Input: dimensioned drawing with shaded views. Units: mm. Origin: part minimum x, y, z. A direction names the side the tool comes from. Round coordinates to 2 decimals unless told otherwise and drop trailing zeros. Order: outer loops, then holes, each group sorted by start corner. A loop starts at its lowest first (then second) coordinate and runs counter-clockwise, first axis right, second up. Notation, with made-up numbers: (-10, -15) - (22, -15) arc R21 ccw to (22, -1) - close; hole circle Ø2 at (49, -18.5). An arc over 180 degrees is marked (long way). Return JSON: item names as keys, results as strings. Group by question number.
1) Contact query for flat-ended pins moving along their axis: P1, Ø1.5, axis at x = 12.5, y = 4, coming from the +Z side; P2, Ø1, axis at x = 54.5, z = 8.5, coming from the -Y side; P3, Ø6, axis at y = 9.5, z = 5, coming from the +X side; P4, Ø7.5, axis at x = 13.5, z = 10, coming from the +Y side. Output: stop coordinate, or through.
2) Access query for the marked faces 4, 5, 6, 7 and 8. Directions: +Z, -Z, +X, -X, +Y, -Y. A direction counts if a zero-diameter tool reaches every point of the face in a straight line with its end or side. Return the directions, or none.
3) Section A-A, the plane x = 88.9. Return loops of the section in (y, z), plus the area to 3 significant figures.
4) Section B-B, the plane y = 3.75. Return loops of the section in (x, z), plus the area to 3 significant figures.
5) Section D-D, the plane x = 73. Return loops of the section in (y, z).
6) Section C-C, the plane z = 22.86. Return loops of the section in (x, y), plus the area to 3 significant figures.
7) Ray query, line 1 (X direction, y = 1, z = 2.54); line 2 (Z direction, x = 88.9, y = 0.9); line 3 (X direction, y = 3.75, z = 12.5). Return the intervals inside material, ascending. Write a range as from..to.
8) Mould query, pull axis X, two halves, no side actions, for the marked faces 1, 2 and 3. Classes: pulls with the +X half, pulls with the -X half, needs draft (parallel to the pull), parting line crosses it, or undercut.
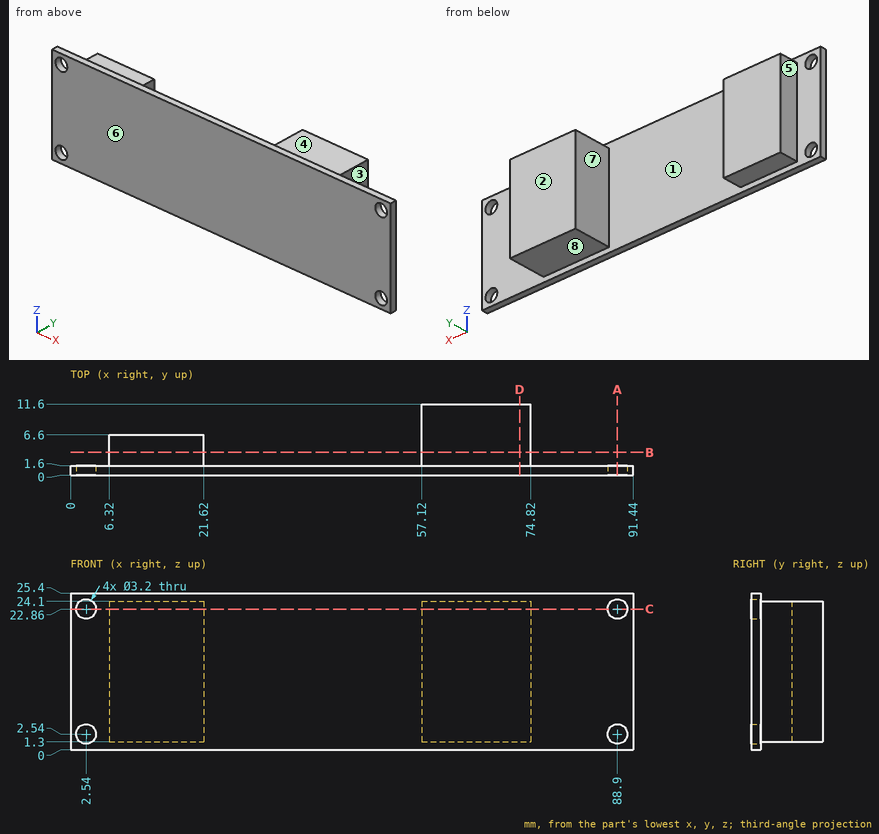
Geometry check:
{
 "1": {"P1": "z = 24.1", "P2": "y = 0", "P3": "x = 74.82", "P4": "y = 6.6"},
 "2": {"face 4": "+Z, +X, -X, +Y", "face 5": "+Z, -Z, -X, +Y", "face 6": "+Z, -Z, +X, -X, -Y", "face 7": "+Z, -Z, +Y", "face 8": "-Z, +X, -X, +Y"},
 "3": {"outline": "(0, 0) - (1.6, 0) - (1.6, 0.94) - (0, 0.94) - close; (0, 4.14) - (1.6, 4.14) - (1.6, 21.26) - (0, 21.26) - close; (0, 24.46) - (1.6, 24.46) - (1.6, 25.4) - (0, 25.4) - close", "area": "30.4 mm2"},
 "4": {"outline": "(6.32, 1.3) - (21.62, 1.3) - (21.62, 24.1) - (6.32, 24.1) - close; (57.12, 1.3) - (74.82, 1.3) - (74.82, 24.1) - (57.12, 24.1) - close", "area": "752 mm2"},
 "5": {"outline": "(0, 0) - (1.6, 0) - (1.6, 1.3) - (11.6, 1.3) - (11.6, 24.1) - (1.6, 24.1) - (1.6, 25.4) - (0, 25.4) - close"},
 "6": {"outline": "(0, 0) - (0.94, 0) - (0.94, 1.6) - (0, 1.6) - close; (4.14, 0) - (87.3, 0) - (87.3, 1.6) - (74.82, 1.6) - (74.82, 11.6) - (57.12, 11.6) - (57.12, 1.6) - (21.62, 1.6) - (21.62, 6.6) - (6.32, 6.6) - (6.32, 1.6) - (4.14, 1.6) - close; (90.5, 0) - (91.44, 0) - (91.44, 1.6) - (90.5, 1.6) - close", "area": "390 mm2"},
 "7": {"line 1": "0..0.94, 4.14..87.3, 90.5..91.44", "line 2": "0..0.94, 4.14..21.26, 24.46..25.4", "line 3": "6.32..21.62, 57.12..74.82"},
 "8": {"face 1": "undercut", "face 2": "needs draft", "face 3": "pulls with the +X half"}
}
